```python
from build123d import *

# Parameters (mm, degrees)
BOSS_EXTRUDE1_DEPTH = 10
SKETCH2_R           = 2.1
CUT_EXTRUDE1_DEPTH  = 5
SKETCH3_R           = 1
CUT_EXTRUDE2_DEPTH  = 13.68857754


with BuildPart() as part:
    # Sketch1 → Boss-Extrude1 (new body)
    with BuildSketch(Plane.XY):
        with BuildLine():
            Line((-6, 3), (6, 3))
            Line((6, 3), (6, -3))
            ThreePointArc((6, -3), (2.579770149, -4.028730546), (0.29453866, -6.77353943))
            ThreePointArc((0.29453866, -6.77353943), (-2.234422316, -3.85538634), (-6, -3))
            Line((-6, -3), (-6, 3))
        make_face()
    extrude(amount=BOSS_EXTRUDE1_DEPTH)

    # Sketch2 → Cut-Extrude1 (cut)
    with BuildSketch(Plane(origin=(0, 3, 0), x_dir=(1, 0, 0), z_dir=(0, 1, 0))):
        with Locations(Location((0, -5, 0), (0, 0, 270))):
            Circle(SKETCH2_R)
    extrude(amount=-CUT_EXTRUDE1_DEPTH, mode=Mode.SUBTRACT)

    # Sketch3 → Cut-Extrude2 (cut, through all)
    with BuildSketch(Plane(origin=(0, -2, 0), x_dir=(1, 0, 0), z_dir=(0, 1, 0))):
        with Locations(Location((0, -5, 0), (0, 0, 270))):
            Circle(SKETCH3_R)
    extrude(amount=-CUT_EXTRUDE2_DEPTH, mode=Mode.SUBTRACT)

    # Boss-Extrude2 cone 1 section (through the dimple's axis) → Boss-Extrude2 (revolve)
    with BuildSketch(Plane(origin=(-4.04459479, -2.85, 5), x_dir=(0, 0, 1), z_dir=(1, 0, 0))):
        Polygon((0, 0), (1.024588898, 0), (0, 1.024588898), align=None)
    revolve(axis=Axis((-4.04459479, -2.85, 5), (0, -1, 0)))


solid = part.part
```
CAD build for the part. Positions are in the model's coordinates, mm. Coordinates: 2 decimals unless noted, no trailing zeros. Order: outer loops, then holes, each group sorted by start corner. A loop starts at its lowest first (then second) coordinate and runs counter-clockwise, first axis right, second up. Notation, with made-up numbers: M 12.25,-36 L 19.25,-36 A28 cw 19.25,-14 Z; hole C 55.25,-18.5 d2. An arc over 180 degrees is marked long. Write each question's results on one line, items separated by ' | '. Start each with the question number.
Q1. Flat gauge pins, fed straight in: P1, Ø1.3, axis at x = 0.5, z = 5, coming from the +Y side; P2, Ø5, axis at x = 4, z = 3.5, coming from the -Y side (3 decimals); P3, Ø1, axis at x = -1, z = 1, coming from the -Y side. Where does each tip first touch, or does it go through?
Q2. Drill centre lines: probe 1 along X at (y, z) = (0.2, 5); probe 2 along Z at (x, y) = (0, -5.15); probe 3 along X at (y, z) = (-3.75, 5). Where is each one in solid material? Low to high. Write a range as from..to.
Q3. Cut at B-B (x = -0.25). List the corners of the cut face in (y, z), then the cut area to 3 significant figures.
Q4. Cut at D-D (y = -3.5). List the corners of the cut face in (x, z), then the cut area to 3 significant figures.
Q5. Cut at A-A (y = 1). List the corners of the cut face in (x, z), then the cut area to 3 significant figures.
Q6. Pull direction Z, two halves, no side cores. Call faces 1 (the flat face through (0, -1, 0)), 2 (the cylindrical face through (1, -4, 5)), 3 (the flat face through (-0.1, 3, 2.7)), 4 (the cylindrical face through (0.09, 0.54, 2.9)): +Z half, -Z half, draft (parallel to the pull), parting line (faces both ways), or undercut.
Q7. Cut at C-C (z = 7.75). List the corners of the cut face in (x, y).
Found:
1) P1: y = -2 | P2: y = -4.935 | P3: y = -5.4
2) probe 1: -6..-2.1, 2.1..6 | probe 2: 0..4, 6..10 | probe 3: -4.17..-3.92, -2.42..-1, 1..3.04
3) outline: M -5.75,0 L 3,0 L 3,2.91 L -2,2.91 L -2,4.03 L -5.75,4.03 Z; M -5.75,5.97 L -2,5.97 L -2,7.09 L 3,7.09 L 3,10 L -5.75,10 Z | area: 59.4 mm²
4) outline: C -4.04,5 d0.75; M -2.92,0 L 3.56,0 L 3.56,10 L -2.92,10 Z; hole C 0,5 d2 | area: 62.1 mm²
5) outline: M -6,0 L 6,0 L 6,10 L -6,10 Z; hole C 0,5 d4.2 | area: 106 mm²
6) face 1: -Z half | face 2: undercut | face 3: draft | face 4: undercut
7) outline: M -6,-3 A6.2 cw 0.29,-6.77 A6.2 cw 6,-3 L 6,3 L -6,3 Z
